For this review, use the dimensioned drawing (mm, ordinates from the lowest corner) and the shaded views. A direction names the side the tool comes from. Give positions to 0.01 mm unless a question says otherwise; leave off trailing zeros. Order: outer loops, then holes, each group sorted by start corner. A loop starts at its lowest first (then second) coordinate and runs counter-clockwise, first axis right, second up. Notation, with made-up numbers: M 63,-36.75 L 97,-36.75 A30 cw 97,-7.75 Z; hole C 6,35.5 d8. An arc over 180 degrees is marked long. Answer as CSV lines item,"result". Start each with the question number.
1. For line 1 along Y through (x, z) = (3.4, 3.15) (1 decimal); line 2 along Z through (x, y) = (3, 8); line 3 along X through (y, z) = (7.75, 1.4) (1 decimal), list the stretches that pass through material, from the lowest coordinate up.
2. We need section B-B, the plane y = 4.5. Give the boundary of the cut face in (x, z).
3. Clearance check with flat-ended pins moving along their axes: P1, Ø0.6, axis at x = 2.5, y = 7.5, coming from the -Z side; P2, Ø1, axis at x = 1.5, y = 7, coming from the +Z side. State where each tip first meets the part, or that it passes through.
4. Machinability: for the marked faces 1, 2 and 3, which of the approach directions +Z, -Z, +X, -X, +Y, -Y give a long, thin tool a straight path to every point of the face, cutting with its end or side? Answer none if there is none.
5. Mouldability with a two-part tool opening along Z and no side actions: class the marked faces 4, 5 and 6 as pulls with the +Z half, pulls with the -Z half, needs draft (parallel to the pull), parting line crosses it, or undercut.
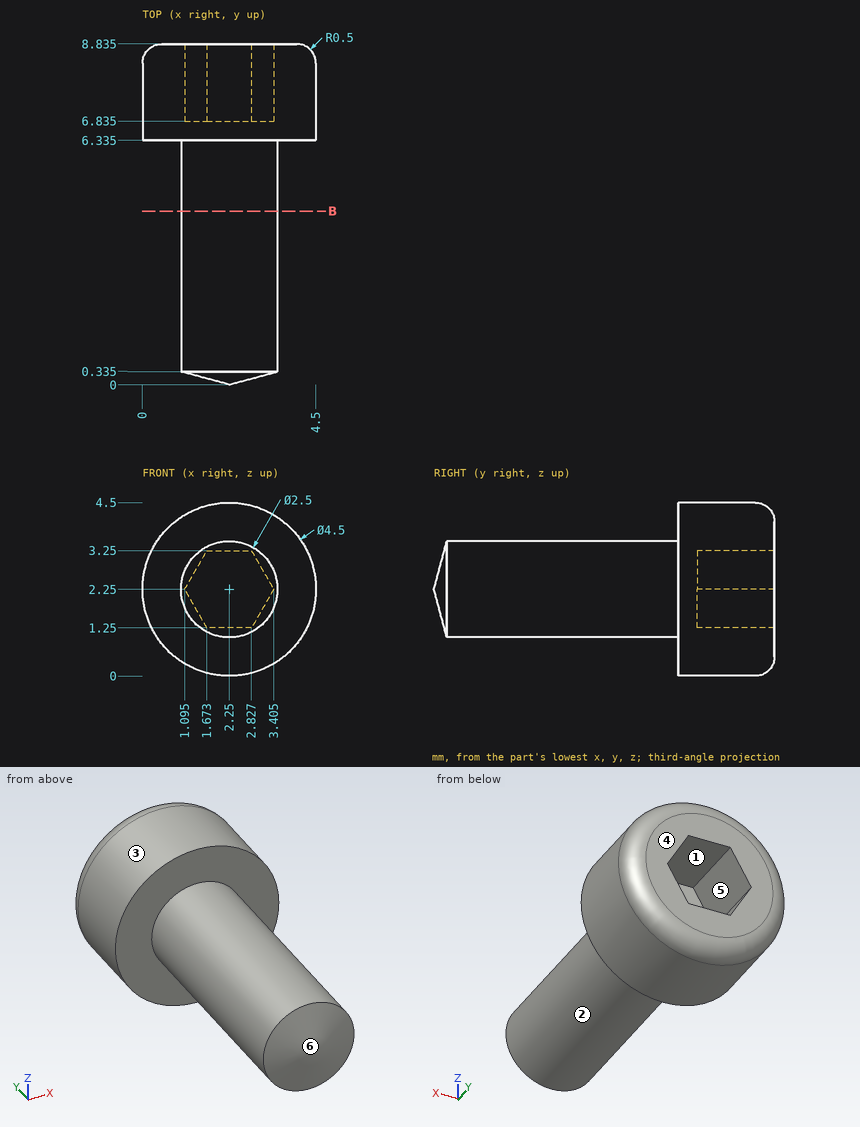
Result set:
1,line 1,"6.3 to 8.8"
1,line 2,"0.13 to 1.55, 2.95 to 4.37"
1,line 3,"0.2 to 1.6, 2.9 to 4.3"
2,outline,"C 2.25,2.25 d2.5"
3,P1,"z = 0"
3,P2,"z = 4.49"
4,face 1,"+Y"
4,face 2,"-Y"
4,face 3,"+Y, -Y"
5,face 4,"needs draft"
5,face 5,"undercut"
5,face 6,"parting line crosses it"
